The model under review builds one solid part; all positions refer to its coordinate system, in mm. Face numbers are marked on the shaded views. A direction names the side the tool comes from. Give positions to 0.01 mm unless a question says otherwise; leave off trailing zeros. Order: outer loops, then holes, each group sorted by start corner. A loop starts at its lowest first (then second) coordinate and runs counter-clockwise, first axis right, second up. Notation, with made-up numbers: (78, 55.25) - (92, 55.25) arc R7 ccw to (92, 63.25) - close; hole circle Ø11 at (-39.5, 89). An arc over 180 degrees is marked (long way). Use a Markdown table: item, result. Add a question column.
Autodesk Inventor part; units mm, degrees
ref_plane "YZ Plane" through (0, 0, 0) normal (1, 0, 0) x (0, 1, 0)
ref_plane "XZ Plane" through (0, 0, 0) normal (0, 1, 0) x (-1, 0, 0)
ref_plane "XY Plane" through (0, 0, 0) normal (0, 0, 1) x (1, 0, 0)
ref_plane "Work Plane1" through (0, 0, 0) normal (0, 0, 1) x (1, 0, 0)
sketch "Sketch1" plane through (0, 0, 0) normal (0, 0, 1) x (1, 0, 0)
  circle A0 centre (173.6996, 946.853) radius 5.5
  circle A1 centre (152.6996, 946.853) radius 5.5
  line L0 (454.025, 962.025) -> (-295.275, 962.025)
  line L1 (-295.275, 962.025) -> (-295.275, -1057.275)
  line L2 (-295.275, -1057.275) -> (454.025, -1057.275)
  line L3 (454.025, -1057.275) -> (454.025, 962.025)
  circle A2 centre (396.1257, -28.5814) radius 31.4325
  line L4 (182.6996, 962.025) -> (142.6996, 962.025)
  line L5 (142.6996, 962.025) -> (142.6996, 929.853)
  line L6 (142.6996, 929.853) -> (182.6996, 929.853)
  line L7 (182.6996, 929.853) -> (182.6996, 962.025)
  line L8 (195.3996, 917.153) -> (129.9996, 917.153)
  line L9 (129.9996, 917.153) -> (129.9996, 974.725)
  line L10 (129.9996, 974.725) -> (195.3996, 974.725)
  line L11 (195.3996, 974.725) -> (195.3996, 917.153)
  point P0 (0, 0)
  point P1 (182.6996, 963.853)
  point P2 (129.9996, 962.025)
  point P3 (195.3996, 962.025)
  dimension "d0" = 12.7
extrude "Extrusion1" add sketch "Sketch1" along normal blind 49.5554 contours L7 L6 L5 L0
extrude "Extrusion2" add sketch "Sketch1" along normal blind 6.35 contours L0 L11 L8 L9 L5 L6 L7
fillet "Fillet1" radius 3.175 5 edges at (182.6996, 945.939, 6.35) (162.6996, 929.853, 6.35) (142.6996, 945.939, 6.35) (142.6996, 929.853, 27.9527) (182.6996, 929.853, 27.9527)
fillet "Fillet2" radius 3.175 2 edges at (129.9996, 962.025, 3.175) (195.3996, 962.025, 3.175)
fillet "Fillet3" radius 15.875 2 edges at (129.9996, 917.153, 3.175) (195.3996, 917.153, 3.175)
properties part number "BracketSpacer"
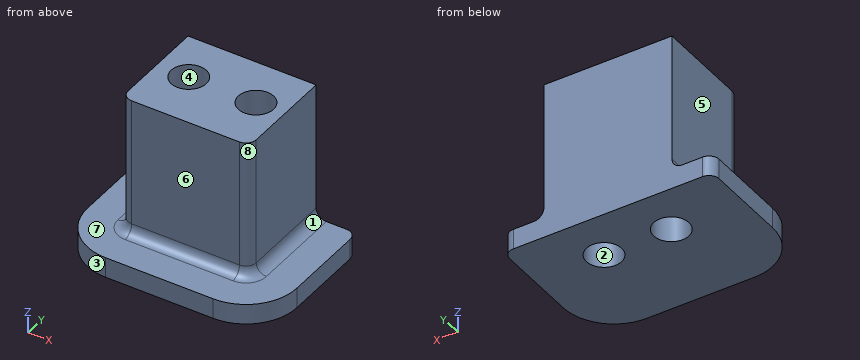
Q1. Machinability: for the marked faces 5, 6, 7 and 8, which of the approach directions +Z, -Z, +X, -X, +Y, -Y give a long, thin tool a straight path to every point of the face, cutting with its end or side? Answer none if there is none.
Q2. Clearance check with flat-ended pins moving along their axes: P1, Ø6, axis at x = 167, z = 38, coming from the -Y side; P2, Ø10, axis at y = 927.5, z = 14.5, coming from the +X side; P3, Ø10, axis at y = 931, z = 36, coming from the -X side. State where each tip first meets the part, or that it passes through.
Q3. Draft analysis for pull direction X (two halves, no side actions). For the marked faces 1, 2, 3 and 4, state which applies: pulls with the +X half, pulls with the -X half, needs draft (parallel to the pull), parting line crosses it, or undercut.
Q4. We need section C-C (z = 5.5). Write out the cut boundary in (x, y) (3 decimals), plus the area to 3 significant figures.
Q5. Wall thickness on probe 1 along X at (y, z) = (948.5, 31); probe 2 along X at (y, z) = (944.5, 47); probe 3 along Z at (x, y) = (172, 922.5): over which ranges is each line inside the solid? List them lowest first.
Q6. We need section A-A (y = 943.5). Write out the cut boundary in (x, z) (3 decimals).
Q7. We need section B-B (y = 934). Write out the cut boundary in (x, z) (3 decimals).
Q8. We need section D-D (x = 163.5). Write out the cut boundary in (y, z) (3 decimals).
Here are the results:
| question | item | result |
|---|---|---|
| 1 | face 5 | +Z, -X, +Y, -Y |
| 1 | face 6 | +Z, +X, -X, -Y |
| 1 | face 7 | +Z, -Y |
| 1 | face 8 | +Z, +X, -Y |
| 2 | P1 | y = 929.85 |
| 2 | P2 | x = 182.66 |
| 2 | P3 | x = 142.7 |
| 3 | face 1 | pulls with the +X half |
| 3 | face 2 | undercut |
| 3 | face 3 | pulls with the -X half |
| 3 | face 4 | undercut |
| 4 | outline | (130, 933.028) arc R15.875 ccw to (145.875, 917.153) - (179.525, 917.153) arc R15.875 ccw to (195.4, 933.028) - (195.4, 958.85) arc R3.175 ccw to (192.225, 962.025) - (133.175, 962.025) arc R3.175 ccw to (130, 958.85) - close; hole circle Ø11 at (152.7, 946.853); hole circle Ø11 at (173.7, 946.853) |
| 4 | area | 2,630 mm2 |
| 5 | probe 1 | 142.7 to 147.45, 157.95 to 168.45, 178.95 to 182.7 |
| 5 | probe 2 | 142.7 to 147.73, 157.67 to 168.73, 178.67 to 182.7 |
| 5 | probe 3 | 0 to 6.35 |
| 6 | outline | (130, 0) - (148.34, 0) - (148.34, 49.555) - (142.7, 49.555) - (142.7, 9.525) arc R3.175 cw to (139.525, 6.35) - (130, 6.35) - close; (157.059, 0) - (169.34, 0) - (169.34, 49.555) - (157.059, 49.555) - close; (178.059, 0) - (195.4, 0) - (195.4, 6.35) - (185.875, 6.35) arc R3.175 cw to (182.7, 9.525) - (182.7, 49.555) - (178.059, 49.555) - close |
| 7 | outline | (130, 0) - (195.4, 0) - (195.4, 6.35) - (185.875, 6.35) arc R3.175 cw to (182.7, 9.525) - (182.7, 49.555) - (142.7, 49.555) - (142.7, 9.525) arc R3.175 cw to (139.525, 6.35) - (130, 6.35) - close |
| 8 | outline | (917.153, 0) - (962.025, 0) - (962.025, 49.555) - (929.853, 49.555) - (929.853, 9.525) arc R3.175 cw to (926.678, 6.35) - (917.153, 6.35) - close |
